The listing builds one solid part. Answer for the finished solid, in the listing's coordinates (mm). A direction names the side the tool comes from. Coordinates: 2 decimals unless noted, no trailing zeros. Loops run counter-clockwise (first coordinate to the right, second up) from the corner with the lowest first, then second, coordinate; pieces in that order, holes last. Notation, with made-up numbers: (61, -26) - (70, -26) arc R22 cw to (70, 4) - close; hole circle Ø7 at (8, 40). An arc over 180 degrees is marked (long way). Return JSON: item names as keys, results as strings. Group by question number.
1. Section B-B (z = 32.5) is taken. Write down the section's boundary in (x, y).
2. The mould has two halves that part along Z. Classify faces 1 (the face through (-81, -1, 0)), 2 (the face through (-79, -1, 50.8)), 3 (the face through (-74.07, -0.78, 3.57)): pulls with the +Z half, pulls with the -Z half, needs draft (parallel to the pull), parting line crosses it, or undercut.
3. Section D-D (x = -71) is taken. Write down the section's boundary in (y, z), and give its area (3 significant figures).
4. Find the intervals of material crossed by line 1 along Z through (x, y) = (-72.5, -3.75); line 2 along Y through (x, z) = (-71, 29.5); line 3 along X through (y, z) = (-12.25, 12), in increasing order.
5. Each of these flat-tipped pins is pushed along its axis until it touches: P1, Ø4.5, axis at x = -106.93, z = 33.53, coming from the -Y side; P2, Ø8, axis at y = -11, z = 11.5, coming from the -X side. Where does it stop, or does it pass through?
6. Which of the six approach directions +Z, -Z, +X, -X, +Y, -Y give full straight-line access (tool end or side, diameter ignored) to faces 4 (the face through (-99.063, -0.783, 21.848)), 5 (the face through (-68, -5, 1.588))?
7. Section C-C (x = -79) is taken. Write down the section's boundary in (y, z), and give its area (3 significant figures).
8. Section A-A (x = -116.5) is taken. Write down the section's boundary in (y, z), and give its area (3 significant figures).
```python
from build123d import *

# Parameters (mm, degrees)
BOSS_EXTRUDE2_DEPTH = 50.8
SKETCH4_R           = 5.05
SKETCH4_R_2         = 4.7625
SKETCH4_R_3         = 1.984375
CUT_EXTRUDE1_DEPTH  = 1.5875
BOSS_EXTRUDE3_DEPTH = 1.5875
BOSS_EXTRUDE4_DEPTH = 1.5875
SKETCH8_R           = 3.175
CUT_EXTRUDE2_DEPTH  = 1.5875


with BuildPart() as part:
    # Sketch3 → Boss-Extrude2 (new body)
    with BuildSketch(Plane.XY):
        Polygon((-121.219673345, 0), (-62.482173345, 0), (-62.482173345, -26.9875), (-64.069673345, -26.9875), (-64.069673345, -1.5875), (-121.219673345, -1.5875), align=None)
    extrude(amount=BOSS_EXTRUDE2_DEPTH)

    # Sketch4 → Cut-Extrude1 (cut)
    with BuildSketch(Plane(origin=(0, 0, 0), x_dir=(1, 0, 0), z_dir=(0, 1, 0))):
        with Locations((-108.519673345, -25.4)):
            Circle(SKETCH4_R)
        with Locations((-79.944673345, -39.2875)):
            Circle(SKETCH4_R_2)
        with Locations((-108.519673345, -15.685)):
            Circle(SKETCH4_R_3)
        with Locations((-87.802397451, -31.429775894)):
            Circle(SKETCH4_R_3)
        with Locations((-72.086949239, -31.429775894)):
            Circle(SKETCH4_R_3)
        with Locations((-72.086949239, -47.145224106)):
            Circle(SKETCH4_R_3)
        with Locations((-87.802397451, -47.145224106)):
            Circle(SKETCH4_R_3)
        with Locations((-116.649673345, -25.4)):
            Circle(SKETCH4_R_3)
        with Locations((-98.804673345, -23.815)):
            Circle(SKETCH4_R_3)
        with Locations((-106.934673345, -33.53)):
            Circle(SKETCH4_R_3)
        with Locations((-87.802397451, -3.654775894)):
            Circle(SKETCH4_R_3)
        with Locations((-72.086949239, -3.654775894)):
            Circle(SKETCH4_R_3)
        with Locations((-72.086949239, -19.370224106)):
            Circle(SKETCH4_R_3)
        with Locations((-87.802397451, -19.370224106)):
            Circle(SKETCH4_R_3)
        with Locations((-79.944673345, -11.5125)):
            Circle(SKETCH4_R_2)
    extrude(amount=-CUT_EXTRUDE1_DEPTH, mode=Mode.SUBTRACT)

    # Sketch5 → Boss-Extrude3 (add)
    with BuildSketch(Plane(origin=(0, 0, 0), x_dir=(-1, 0, 0), z_dir=(0, 0, -1))):
        Polygon((76.769673345, -1.5875), (64.069673345, -14.2875), (64.069673345, -1.5875), align=None)
    extrude(amount=-BOSS_EXTRUDE3_DEPTH)

    # Sketch7 → Boss-Extrude4 (add)
    with BuildSketch(Plane.XY.offset(50.8)):
        Polygon((-64.069673345, -1.5875), (-64.069673345, -14.2875), (-76.769673345, -1.5875), align=None)
    extrude(amount=-BOSS_EXTRUDE4_DEPTH)

    # Sketch8 → Cut-Extrude2 (cut)
    with BuildSketch(Plane(origin=(-62.482173345, 0, 0), x_dir=(0, 0, -1), z_dir=(1, 0, 0))):
        with Locations((-44.45, -18.725361779)):
            Circle(SKETCH8_R)
        with Locations((-6.35, -18.725361779)):
            Circle(SKETCH8_R)
    extrude(amount=-CUT_EXTRUDE2_DEPTH, mode=Mode.SUBTRACT)


solid = part.part
```
The answers:
{
 "1": {"outline": "(-121.22, -1.59) - (-108.63, -1.59) - (-108.63, 0) - (-121.22, 0) - close; (-105.24, -1.59) - (-89.47, -1.59) - (-89.47, 0) - (-105.24, 0) - close; (-86.13, -1.59) - (-73.76, -1.59) - (-73.76, 0) - (-86.13, 0) - close; (-70.42, -1.59) - (-64.07, -1.59) - (-64.07, -26.99) - (-62.48, -26.99) - (-62.48, 0) - (-70.42, 0) - close"},
 "2": {"face 1": "pulls with the -Z half", "face 2": "pulls with the +Z half", "face 3": "undercut"},
 "3": {"outline": "(-7.36, 0) - (0, 0) - (0, 1.99) - (-1.59, 1.99) - (-1.59, 1.59) - (-7.36, 1.59) - close; (-7.36, 49.21) - (-1.59, 49.21) - (-1.59, 48.81) - (0, 48.81) - (0, 50.8) - (-7.36, 50.8) - close; (-1.59, 5.31) - (0, 5.31) - (0, 17.71) - (-1.59, 17.71) - close; (-1.59, 21.03) - (0, 21.03) - (0, 29.77) - (-1.59, 29.77) - close; (-1.59, 33.09) - (0, 33.09) - (0, 45.49) - (-1.59, 45.49) - close", "area": "77.9 mm2"},
 "4": {"line 1": "z = 0 to 1.59, 49.21 to 50.8", "line 2": "y = -1.59 to 0", "line 3": "x = -64.07 to -62.48"},
 "5": {"P1": "stops at y = -1.59", "P2": "stops at x = -64.07"},
 "6": {"face 4": "+Y, -Y", "face 5": "-X, -Y"},
 "7": {"outline": "(-1.59, 0) - (0, 0) - (0, 6.84) - (-1.59, 6.84) - close; (-1.59, 16.18) - (0, 16.18) - (0, 34.62) - (-1.59, 34.62) - close; (-1.59, 43.96) - (0, 43.96) - (0, 50.8) - (-1.59, 50.8) - close", "area": "51.0 mm2"},
 "8": {"outline": "(-1.59, 0) - (0, 0) - (0, 23.42) - (-1.59, 23.42) - close; (-1.59, 27.38) - (0, 27.38) - (0, 50.8) - (-1.59, 50.8) - close", "area": "74.4 mm2"}
}
